For this review, take the finished solid that the model builds, in its own axes (mm). Face numbers are marked on the shaded views. Give positions to 0.01 mm unless a question says otherwise; leave off trailing zeros. Order: outer loops, then holes, each group sorted by start corner. A loop starts at its lowest first (then second) coordinate and runs counter-clockwise, first axis right, second up. Notation, with made-up numbers: (8, -39) - (41, -39) arc R21 cw to (41, -29) - close; hole circle Ø5 at (-12.75, 17). An arc over 180 degrees is marked (long way). Answer as a JSON object with one key per item and string values. Group by question number.
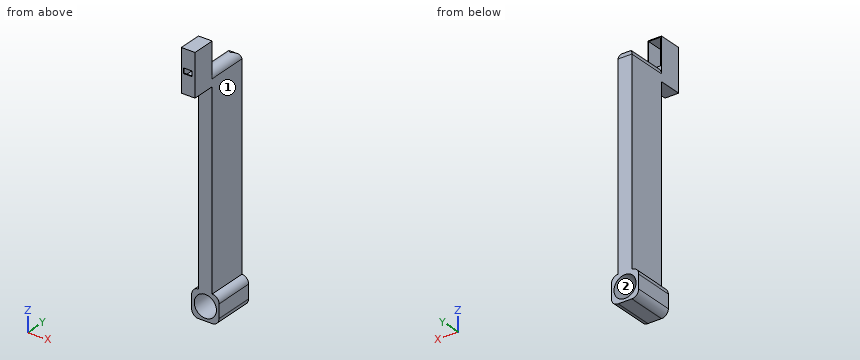
from build123d import *

# Parameters (mm, degrees)
SKETCH2_W           = 34
SKETCH2_H           = 512
SKETCH2_H_2         = 70
SKETCH2_W_2         = 68
SKETCH2_H_3         = 68
BOSS_EXTRUDE1_DEPTH = 158
FILLET1_R           = 17
SKETCH3_W           = 599.373930515
SKETCH3_H           = 58
CUT_EXTRUDE1_DEPTH  = 158
SKETCH4_W           = 68
SKETCH4_H           = 58
CUT_EXTRUDE2_DEPTH  = 158
SKETCH5_R           = 27.5
CUT_EXTRUDE3_DEPTH  = 158
SKETCH6_W           = 70
SKETCH6_H           = 100
CUT_EXTRUDE4_DEPTH  = 84
SKETCH7_W           = 30
SKETCH7_H           = 66
CUT_EXTRUDE6_DEPTH  = 56
SKETCH8_W           = 22
SKETCH8_H           = 13
CUT_EXTRUDE7_DEPTH  = 56
FILLET2_R           = 17
SKETCH9_W           = 455
SKETCH9_H           = 70
CUT_EXTRUDE8_DEPTH  = 111
SKETCH10_W          = 470.461866989
SKETCH10_H          = 86.836519433
BOSS_EXTRUDE3_DEPTH = 34


# Some blends are built 0.0001 mm under size
with BuildPart() as part:
    # Sketch2 → Boss-Extrude1 (new body)
    with BuildSketch(Plane(origin=(0, 0, 0), x_dir=(1, 0, 0), z_dir=(0, 1, 0))):
        with Locations((-34, -324)):
            Rectangle(SKETCH2_W, SKETCH2_H)
        with Locations((-34, -615)):
            Rectangle(SKETCH2_W, SKETCH2_H_2)
        with Locations((-34, -34)):
            Rectangle(SKETCH2_W_2, SKETCH2_H_3)
    extrude(amount=BOSS_EXTRUDE1_DEPTH)

    # Fillet1
    fillet1_edges = [part.edges().sort_by_distance(p)[0] for p in [
        (0, 79, 0),
        (0, 79, 68),
        (-68, 79, 0),
        (-68, 79, 68),
    ]]
    fillet(fillet1_edges, radius=FILLET1_R - 0.0001)  # a hair under: the kernel refuses the full size

    # Sketch3 → Cut-Extrude1 (cut)
    with BuildSketch(Plane.ZY.offset(51)):
        with Locations((245.313034743, 29)):
            Rectangle(SKETCH3_W, SKETCH3_H)
    extrude(amount=-CUT_EXTRUDE1_DEPTH, mode=Mode.SUBTRACT)

    # Sketch4 → Cut-Extrude2 (cut)
    with BuildSketch(Plane(origin=(-51, 0, 0), x_dir=(0, 0, -1), z_dir=(1, 0, 0))):
        with Locations((-34, 29)):
            Rectangle(SKETCH4_W, SKETCH4_H)
    extrude(amount=-CUT_EXTRUDE2_DEPTH, mode=Mode.SUBTRACT)

    # Sketch5 → Cut-Extrude3 (cut)
    with BuildSketch(Plane(origin=(0, 158, 0), x_dir=(1, 0, 0), z_dir=(0, 1, 0))):
        with Locations(Location((-34, -34, 0), (0, 0, 270))):
            Circle(SKETCH5_R)
    extrude(amount=-CUT_EXTRUDE3_DEPTH, mode=Mode.SUBTRACT)

    # Sketch6 → Cut-Extrude4 (cut)
    with BuildSketch(Plane.ZY.offset(51)):
        with Locations((615, 108)):
            Rectangle(SKETCH6_W, SKETCH6_H)
    extrude(amount=-CUT_EXTRUDE4_DEPTH, mode=Mode.SUBTRACT)

    # Sketch7 → Cut-Extrude6 (cut)
    with BuildSketch(Plane(origin=(0, 58, 0), x_dir=(1, 0, 0), z_dir=(0, 1, 0))):
        with Locations((-34, -615)):
            Rectangle(SKETCH7_W, SKETCH7_H)
    extrude(amount=-CUT_EXTRUDE6_DEPTH, mode=Mode.SUBTRACT)

    # Sketch8 → Cut-Extrude7 (cut)
    with BuildSketch(Plane(origin=(0, 2, 0), x_dir=(1, 0, 0), z_dir=(0, 1, 0))):
        with Locations((-35, -598.5)):
            Rectangle(SKETCH8_W, SKETCH8_H)
    extrude(amount=-CUT_EXTRUDE7_DEPTH, mode=Mode.SUBTRACT)

    # Fillet2
    # the kernel refuses this fillet: 17 mm, written as the material it adds along each edge
    # the kernel refuses this fillet: 17 mm, written as the material it takes off along each edge
    with BuildSketch(Plane(origin=(-93.5, 158, 580), x_dir=(0, 0, -1), z_dir=(1, 0, 0))) as fillet2_2_piece_1:
        with BuildLine():
            CenterArc((FILLET2_R, -FILLET2_R), FILLET2_R, 90, 90)
            Line((0, -FILLET2_R), (0, 0))
            Line((0, 0), (FILLET2_R, 0))
        make_face()
    extrude(amount=119, mode=Mode.SUBTRACT)
    with BuildSketch(Plane(origin=(-17, 200.5, 580), x_dir=(0, 0, -1), z_dir=(0, -1, 0))) as fillet2_2_piece_2:
        with BuildLine():
            CenterArc((FILLET2_R, -FILLET2_R), FILLET2_R, 90, 90)
            Line((0, -FILLET2_R), (0, 0))
            Line((0, 0), (FILLET2_R, 0))
        make_face()
    extrude(amount=142.5, mode=Mode.SUBTRACT)
    with BuildSketch(Plane(origin=(-51, 200.5, 580), x_dir=(0, 0, -1), z_dir=(0, -1, 0))) as fillet2_2_piece_3:
        with BuildLine():
            CenterArc((FILLET2_R, FILLET2_R), FILLET2_R, 180, 90)
            Line((0, FILLET2_R), (0, 0))
            Line((0, 0), (FILLET2_R, 0))
        make_face()
    extrude(amount=142.5, mode=Mode.SUBTRACT)

    # Sketch9 → Cut-Extrude8 (cut)
    with BuildSketch(Plane(origin=(-17, 0, 0), x_dir=(0, 0, -1), z_dir=(1, 0, 0))):
        with Locations((-315.5, 108)):
            Rectangle(SKETCH9_W, SKETCH9_H)
    extrude(amount=-CUT_EXTRUDE8_DEPTH, mode=Mode.SUBTRACT)

    # Sketch10 → Boss-Extrude3 (add)
    with BuildSketch(Plane.ZY.offset(51)):
        with Locations((313.691639381, 107.94529393)):
            Rectangle(SKETCH10_W, SKETCH10_H)
    extrude(amount=-BOSS_EXTRUDE3_DEPTH)


solid = part.part
1) Mouldability with a two-part tool opening along Z and no side actions: class the marked faces 1 and 2 as released by +Z, released by -Z, zero draft, split by the parting line, or undercut.
2) Consider section A-A (x = -34). Give the boundary of the cut face in (y, z).
3) Consider section D-D (y = 33). Give the boundary of the cut face in (x, z), plus the area to 3 significant figures.
4) For pin 1 (17 mm diameter, centred on y = 38.5, z = 615, fed in from +X); pin 2 (12 mm diameter, centred on x = -61, z = 567.5, fed in from -Y); pin 3 (3 mm diameter, centred on x = -18, y = 53, fed in from -Z); pin 4 (15 mm diameter, centred on x = -31.5, z = 609, fed in from +Y), all flat-tipped, find the tip position at first contact; note any pin that passes through.
5) For line 1 (X direction, y = 125.5, z = 34); line 2 (Z direction, x = -41, y = 20); line 3 (Y direction, x = -43.5, z = 152), list the stretches that pass through material, from the lowest coordinate up.
6) Consider section C-C (z = 34). Give the boundary of the cut face in (x, y).
Result set:
{
 "1": {"face 1": "zero draft", "face 2": "undercut"},
 "2": {"outline": "(0, 545) - (58, 545) - (58, 61.5) - (158, 61.5) - (158, 563) arc R17 ccw to (141, 580) - (58, 580) - (58, 582) - (2, 582) - (2, 592) - (0, 592) - close; (0, 605) - (2, 605) - (2, 648) - (58, 648) - (58, 650) - (0, 650) - close; (58, 0) - (158, 0) - (158, 6.5) - (58, 6.5) - close"},
 "3": {"outline": "(-51, 545) - (-17, 545) - (-17, 650) - (-51, 650) - close; hole (-49, 582) - (-19, 582) - (-19, 648) - (-49, 648) - close", "area": "1,590 mm2"},
 "4": {"pin 1": "stops at x = -17", "pin 2": "passes through", "pin 3": "stops at z = 545", "pin 4": "stops at y = 2"},
 "5": {"line 1": "x = -68 to -61.5, -6.5 to 0", "line 2": "z = 545 to 582, 648 to 650", "line 3": "y = 58 to 158"},
 "6": {"outline": "(-68, 58) - (-61.5, 58) - (-61.5, 158) - (-68, 158) - close; (-6.5, 58) - (0, 58) - (0, 158) - (-6.5, 158) - close"}
}
